For this review, take the finished solid that the model builds, in its own axes (mm). A direction names the side the tool comes from. Give positions to 0.01 mm unless a question says otherwise; leave off trailing zeros. Order: outer loops, then holes, each group sorted by start corner. A loop starts at its lowest first (then second) coordinate and runs counter-clockwise, first axis right, second up. Notation, with made-up numbers: (48, 15) -> (64, 15) arc R22 cw to (64, 22) -> close; hole circle Ø6 at (16.5, -29.75). An arc over 180 degrees is marked (long way). Return JSON: item names as keys, results as strings. Group by question number.
1) Add section B-B (x = 49). Give the boundary of the cut face in (y, z), then the cut area to 3 significant figures.
2) Add section D-D (x = 23.1). Give the boundary of the cut face in (y, z).
3) The part is to be moulded in two halves that separate along Y. For faces 4 (the face through (84, 7, -57)), 5 (the face through (0, 13, -59)), 6 (the face through (5, 15, -5)), say which applies: released by +Y, released by -Y, zero draft, split by the parting line, or undercut.
4) Add section A-A (y = 4). Give the boundary of the cut face in (x, z).
5) For faces 1 (the face through (1.014, 12.626, -24.099)), 2 (the face through (5, 15, -115)), 3 (the face through (4.921, 22.056, -3.165)), list the 3-axis set-ups (+Z, -Z, +X, -X, +Y, -Y) from which the entire face can be reached by the end or side of a thin tool; tool diameter is ignored.
6) To check wall thickness, follow line 1 along Z through (x, y) = (105.5, 20); line 2 along X through (y, z) = (22.5, -115.5); line 3 along X through (y, z) = (18, -77.5). State the ranges of each line that lie inside material, in increasing order.
7) Add section C-C (z = -39). Give the boundary of the cut face in (x, y).
8) Insertion check: P1, Ø6.5, axis at x = 49, y = 23, coming from the +Z side; P2, Ø2, axis at x = 20.5, z = -54.5, coming from the +Y side; P3, Ø8, axis at x = 39, z = -96, coming from the +Y side. Each pin has a flat end and moves straight along its axis. Give the tip position at first contact, or say it passes through.
from build123d import *
from OCP.BRepFilletAPI import BRepFilletAPI_MakeChamfer

# Parameters (mm, degrees)
SKETCH_1_W                = 110
SKETCH_1_H                = 120
EXTRUDE_1_DEPTH           = 2
SKETCH_2_R                = 5
EXTRUDE_2_DEPTH           = 5
EXTRUDE_2_DRAFT           = 15
EXTRUDE_2_PROFILE_2_DEPTH = 5
EXTRUDE_2_PROFILE_2_DRAFT = 15
EXTRUDE_2_PROFILE_3_DEPTH = 5
EXTRUDE_2_PROFILE_3_DRAFT = 15
SKETCH_3_R                = 1.4
CUT_EXTRUDE_1_DEPTH       = 5
SKETCH_4_W                = 110
SKETCH_4_H                = 120
SKETCH_4_W_2              = 106
SKETCH_4_H_2              = 116
EXTRUDE_3_DEPTH           = 24
SKETCH_5_W                = 6
SKETCH_5_H                = 6
EXTRUDE_4_DEPTH           = 8
CHAMFER_1_SIZE            = 6
SKETCH_6_R                = 1.4
CUT_EXTRUDE_2_DEPTH       = 8
FILLET_1_R                = 3
CHAMFER_2_SIZE            = 0.4
CHAMFER_3_SIZE            = 0.4
CHAMFER_3_SIZE2           = 0.565685425
SKETCH_8_R                = 4
CUT_EXTRUDE_3_DEPTH       = 3
FILLET_2_R                = 0.4
SKETCH_9_R                = 3.25
CUT_EXTRUDE_4_DEPTH       = 10
SKETCH_10_R               = 1.75
CUT_EXTRUDE_5_DEPTH       = 10


with BuildPart() as part:
    # 草图1 → 凸台-拉伸1 (new body)
    with BuildSketch(Plane(origin=(0, 0, 0), x_dir=(1, 0, 0), z_dir=(0, 1, 0))):
        with Locations((55, 60)):
            Rectangle(SKETCH_1_W, SKETCH_1_H)
    extrude(amount=EXTRUDE_1_DEPTH)


with BuildPart() as extrude_2_tool:
    # 草图2 → 凸台-拉伸2 (with draft: the straight prism first)
    with BuildSketch(Plane(origin=(0, 2, 0), x_dir=(1, 0, 0), z_dir=(0, 1, 0))):
        with Locations((82.1, 56.57)):
            Circle(SKETCH_2_R)
    extrude(amount=EXTRUDE_2_DEPTH)
    # 凸台-拉伸2: the draft: its side faces are tilted about the plane it starts from
    extrude_2_sides = [extrude_2_tool.faces().sort_by_distance(p)[0] for p in [
        (77.1, 4.5, -56.57),
    ]]
    draft(extrude_2_sides, Plane(origin=(0, 2, 0), x_dir=(1, 0, 0), z_dir=(0, 1, 0)), EXTRUDE_2_DRAFT)


with BuildPart() as part_1:
    add(part.part)

    # 凸台-拉伸2: add extrude_2_tool
    add(extrude_2_tool.part)


with BuildPart() as extrude_2_profile_2_tool:
    # 草图2 → 凸台-拉伸2 profile 2 (with draft: the straight prism first)
    with BuildSketch(Plane(origin=(0, 2, 0), x_dir=(1, 0, 0), z_dir=(0, 1, 0))):
        with Locations((38.1, 94.57)):
            Circle(SKETCH_2_R)
    extrude(amount=EXTRUDE_2_PROFILE_2_DEPTH)
    # 凸台-拉伸2 profile 2: the draft: its side faces are tilted about the plane it starts from
    extrude_2_profile_2_sides = [extrude_2_profile_2_tool.faces().sort_by_distance(p)[0] for p in [
        (33.1, 4.5, -94.57),
    ]]
    draft(extrude_2_profile_2_sides, Plane(origin=(0, 2, 0), x_dir=(1, 0, 0), z_dir=(0, 1, 0)), EXTRUDE_2_PROFILE_2_DRAFT)


with BuildPart() as part_2:
    add(part_1.part)

    # 凸台-拉伸2 profile 2: add extrude_2_profile_2_tool
    add(extrude_2_profile_2_tool.part)


with BuildPart() as extrude_2_profile_3_tool:
    # 草图2 → 凸台-拉伸2 profile 3 (with draft: the straight prism first)
    with BuildSketch(Plane(origin=(0, 2, 0), x_dir=(1, 0, 0), z_dir=(0, 1, 0))):
        with Locations((23.1, 13.57)):
            Circle(SKETCH_2_R)
    extrude(amount=EXTRUDE_2_PROFILE_3_DEPTH)
    # 凸台-拉伸2 profile 3: the draft: its side faces are tilted about the plane it starts from
    extrude_2_profile_3_sides = [extrude_2_profile_3_tool.faces().sort_by_distance(p)[0] for p in [
        (18.1, 4.5, -13.57),
    ]]
    draft(extrude_2_profile_3_sides, Plane(origin=(0, 2, 0), x_dir=(1, 0, 0), z_dir=(0, 1, 0)), EXTRUDE_2_PROFILE_3_DRAFT)


with BuildPart() as part_3:
    add(part_2.part)

    # 凸台-拉伸2 profile 3: add extrude_2_profile_3_tool
    add(extrude_2_profile_3_tool.part)

    # 草图3 → 切除-拉伸1 (cut)
    with BuildSketch(Plane(origin=(0, 7, 0), x_dir=(1, 0, 0), z_dir=(0, 1, 0))):
        with Locations(Location((82.1, 56.57, 0), (0, 0, 270))):
            Circle(SKETCH_3_R)
        with Locations(Location((38.1, 94.57, 0), (0, 0, 270))):
            Circle(SKETCH_3_R)
        with Locations(Location((23.1, 13.57, 0), (0, 0, 270))):
            Circle(SKETCH_3_R)
    extrude(amount=-CUT_EXTRUDE_1_DEPTH, mode=Mode.SUBTRACT)

    # 草图4 → 凸台-拉伸3 (add)
    with BuildSketch(Plane(origin=(0, 2, 0), x_dir=(1, 0, 0), z_dir=(0, 1, 0))):
        with Locations((55, 60)):
            Rectangle(SKETCH_4_W, SKETCH_4_H)
        with Locations((55, 60)):
            Rectangle(SKETCH_4_W_2, SKETCH_4_H_2, mode=Mode.SUBTRACT)
    extrude(amount=EXTRUDE_3_DEPTH)

    # 草图5 → 凸台-拉伸4 (add)
    with BuildSketch(Plane(origin=(0, 26, 0), x_dir=(1, 0, 0), z_dir=(0, 1, 0))):
        with Locations((5, 115)):
            Rectangle(SKETCH_5_W, SKETCH_5_H)
        with Locations((105, 115)):
            Rectangle(SKETCH_5_W, SKETCH_5_H)
        with Locations((105, 5)):
            Rectangle(SKETCH_5_W, SKETCH_5_H)
        with Locations((5, 5)):
            Rectangle(SKETCH_5_W, SKETCH_5_H)
    extrude(amount=-EXTRUDE_4_DEPTH)

    # 倒角1
    chamfer_1_edges = [part_3.edges().sort_by_distance(p)[0] for p in [
        (105, 18, -118),
        (5, 18, -118),
        (105, 18, -2),
        (5, 18, -2),
    ]]
    chamfer(chamfer_1_edges, length=CHAMFER_1_SIZE - 0.0001)  # a hair under: the kernel refuses the full size

    # 草图6 → 切除-拉伸2 (cut)
    with BuildSketch(Plane(origin=(0, 26, 0), x_dir=(1, 0, 0), z_dir=(0, 1, 0))):
        with Locations(Location((4.5, 115.5, 0), (0, 0, 270))):
            Circle(SKETCH_6_R)
        with Locations(Location((105.5, 115.5, 0), (0, 0, 270))):
            Circle(SKETCH_6_R)
        with Locations(Location((105.5, 4.5, 0), (0, 0, 270))):
            Circle(SKETCH_6_R)
        with Locations(Location((4.5, 4.5, 0), (0, 0, 270))):
            Circle(SKETCH_6_R)
    extrude(amount=-CUT_EXTRUDE_2_DEPTH, mode=Mode.SUBTRACT)

    # 圆角1
    fillet_1_edges = [part_3.edges().sort_by_distance(p)[0] for p in [
        (8, 22, -8),
        (8, 22, -112),
        (102, 22, -112),
        (0, 13, -120),
        (110, 13, -120),
        (110, 13, 0),
        (0, 13, 0),
        (102, 22, -8),
    ]]
    fillet(fillet_1_edges, radius=FILLET_1_R)

    # 倒角2
    chamfer_2_edges = [part_3.edges().sort_by_distance(p)[0] for p in [
        (55, 0, 0),
        (0, 0, -60),
        (55, 0, -120),
        (110, 0, -60),
        (0.878679656, 0, -119.121320344),
        (109.121320344, 0, -119.121320344),
        (109.121320344, 0, -0.878679656),
        (0.878679656, 0, -0.878679656),
    ]]
    chamfer(chamfer_2_edges, length=CHAMFER_2_SIZE)

    # 倒角3: one chamfer whose edges measure the first distance from different faces: ONE call of the kernel's chamfer builder (chamfer() names one face for all edges)
    chamfer_3_edges_1 = [part_3.edges().sort_by_distance(p)[0] for p in [
        (2, 7.00005, -118),
        (108, 7.00005, -118),
        (108, 7.00005, -2),
        (2, 7.00005, -2),
        (55, 2, -118),
        (2, 2, -60),
        (55, 2, -2),
        (108, 2, -60),
    ]]
    chamfer_3_edges_2 = [part_3.edges().sort_by_distance(p)[0] for p in [
        (77.1, 2, -56.57),
        (33.1, 2, -94.57),
        (18.1, 2, -13.57),
    ]]
    chamfer_3_side_2 = [part_3.faces().sort_by_distance(p)[0] for p in [
        (55.141315111, 2, -60.099571799),
    ]]
    chamfer_3 = BRepFilletAPI_MakeChamfer(part_3.part.solid().wrapped)
    for e in chamfer_3_edges_1:
        chamfer_3.Add(CHAMFER_3_SIZE, e.wrapped)
    for e in chamfer_3_edges_2:
        chamfer_3.Add(CHAMFER_3_SIZE, CHAMFER_3_SIZE2, e.wrapped, chamfer_3_side_2[0].wrapped)  # the first distance lies on this face
    add(Compound.cast(chamfer_3.Shape()), mode=Mode.REPLACE)

    # 草图8 → 切除-拉伸3 (cut)
    with BuildSketch(Plane.XY):
        with Locations((49, 23)):
            Circle(SKETCH_8_R)
    extrude(amount=-CUT_EXTRUDE_3_DEPTH, mode=Mode.SUBTRACT)

    # 圆角2
    fillet_2_edges = [part_3.edges().sort_by_distance(p)[0] for p in [
        (46.354248689, 26, -1),
        (51.645751311, 26, -1),
    ]]
    fillet(fillet_2_edges, radius=FILLET_2_R)

    # 草图9 → 切除-拉伸4 (cut)
    with BuildSketch(Plane.ZY.offset(-108)):
        with Locations((-94, 16)):
            Circle(SKETCH_9_R)
    extrude(amount=-CUT_EXTRUDE_4_DEPTH, mode=Mode.SUBTRACT)

    # 草图10 → 切除-拉伸5 (cut)
    with BuildSketch(Plane(origin=(2, 0, 0), x_dir=(0, 0, -1), z_dir=(1, 0, 0))):
        with Locations((22.430011451, 12.100047346)):
            Circle(SKETCH_10_R)
        with Locations((17.350013958, 12.100047346)):
            Circle(SKETCH_10_R)
    extrude(amount=-CUT_EXTRUDE_5_DEPTH, mode=Mode.SUBTRACT)


solid = part_3.part
Evaluation:
{
 "1": {"outline": "(0, -119.6) -> (0.4, -120) -> (26, -120) -> (26, -118) -> (2.4, -118) -> (2, -117.6) -> (2, -2.4) -> (2.4, -2) -> (19, -2) -> (19, 0) -> (0.4, 0) -> (0, -0.4) -> close", "area": "322 mm^2"},
 "2": {"outline": "(0, -119.6) -> (0.4, -120) -> (26, -120) -> (26, -118) -> (2.4, -118) -> (2, -117.6) -> (2, -18.97) -> (2.55, -18.42) -> (7, -17.23) -> (7, -14.97) -> (2, -14.97) -> (2, -12.17) -> (7, -12.17) -> (7, -9.91) -> (2.55, -8.72) -> (2, -8.17) -> (2, -2.4) -> (2.4, -2) -> (26, -2) -> (26, 0) -> (0.4, 0) -> (0, -0.4) -> close"},
 "3": {"face 4": "released by +Y", "face 5": "zero draft", "face 6": "undercut"},
 "4": {"outline": "(0, -117) arc R3 ccw to (3, -120) -> (107, -120) arc R3 ccw to (110, -117) -> (110, -3) arc R3 ccw to (107, 0) -> (3, 0) arc R3 ccw to (0, -3) -> close; circle Ø8.93 at (23.1, -13.57); circle Ø8.93 at (38.1, -94.57); circle Ø8.93 at (82.1, -56.57); hole (2, -117.6) -> (2.4, -118) -> (107.6, -118) -> (108, -117.6) -> (108, -2.4) -> (107.6, -2) -> (2.4, -2) -> (2, -2.4) -> close; hole circle Ø2.8 at (23.1, -13.57); hole circle Ø2.8 at (38.1, -94.57); hole circle Ø2.8 at (82.1, -56.57)"},
 "5": {"face 1": "-X", "face 2": "none", "face 3": "+Y"},
 "6": {"line 1": "-120 to -116.9, -114.1 to -112, -8 to -5.9, -3.1 to 0", "line 2": "0 to 3.1, 5.9 to 8, 102 to 104.1, 106.9 to 110", "line 3": "0 to 2, 108 to 110"},
 "7": {"outline": "(0, 0.4) -> (0.4, 0) -> (109.6, 0) -> (110, 0.4) -> (110, 26) -> (108, 26) -> (108, 2.4) -> (107.6, 2) -> (2.4, 2) -> (2, 2.4) -> (2, 26) -> (0, 26) -> close"},
 "8": {"P1": "z = -118", "P2": "y = 2", "P3": "y = 7"}
}
